Check sheet for the modelled part. Datum: model origin and axes. Units: mm. A direction names the side the tool comes from. Give positions to 0.01 mm unless a question says otherwise; leave off trailing zeros. Order: outer loops, then holes, each group sorted by start corner. A loop starts at its lowest first (then second) coordinate and runs counter-clockwise, first axis right, second up.
Item 1: Sectioned sample at C-C on z = 3.25. Record the boundary of the cut face in (x, y).
Item 2: Access from +Z, -Z, +X, -X, +Y, -Y to the whole of each face (thin tool, end or side, straight path). Record for faces 1 (the cylindrical face through (-1.952, 2.465, -1.864)), 2 (the flat face through (0, 6.35, 1)), 3 (the flat face through (1, 2.5, 2)).
Item 3: Sectioned sample at B-B on z = -1.43. Record the boundary of the cut face in (x, y), and give its area (3 significant figures).
Item 4: Material ranges on line 1 along X through (y, z) = (0.75, 0.75); line 2 along X through (y, z) = (2, -1.5); line 3 along X through (y, z) = (5.7, -1.43), recorded low to high.
Item 5: Sectioned sample at D-D on y = 3. Record the boundary of the cut face in (x, z).
Item 6: Gauge pin test, flat ends, axial feed: P1, Ø1.5, axis at x = -0.5, z = -0.5, coming from the -Y side; P2, Ø2.5, axis at x = 0, z = -1.43, coming from the -Y side. Record the tip position at first contact, or that the pin passes through.
Item 7: Sectioned sample at A-A on x = 0. Record the boundary of the cut face in (y, z), and give its area (3 significant figures).
Item 8: Release check for a two-part mould opening along X. For faces 4 (the flat face through (1.77, 1, 2)), 5 (the flat face through (2.16, 3, 0)), 6 (the flat face through (0, 0, 2)) record: released by +X, released by -X, zero draft, split by the parting line, or undercut.
from build123d import *

# Parameters (mm, degrees)
SKETCH_1_W          = 4.32
SKETCH_1_H          = 7.3
SKETCH_1_R          = 2
SKETCH_1_R_2        = 1.5
EXTRUDE_2_DEPTH     = 6.35
SKETCH_1_4_R        = 2
SKETCH_1_4_R_2      = 1.5
CUT_EXTRUDE_1_DEPTH = 5
SKETCH_2_W          = 1
SKETCH_2_H          = 4.148817955
CUT_EXTRUDE_2_DEPTH = 2.5


with BuildPart() as part:
    # Sketch 1 → Extrude 2 (new body)
    # profile 1 of 2: a face of its own
    with BuildSketch(Plane(origin=(0, 0, 0), x_dir=(1, 0, 0), z_dir=(0, 1, 0))):
        Rectangle(SKETCH_1_W, SKETCH_1_H)
        with Locations((0, 1.43)):
            Circle(SKETCH_1_R, mode=Mode.SUBTRACT)
    # profile 2 of 2: a face of its own
    with BuildSketch(Plane(origin=(0, 0, 0), x_dir=(1, 0, 0), z_dir=(0, 1, 0))):
        with Locations((0, 1.43)):
            Circle(SKETCH_1_R)
        with Locations(Location((0, 1.43, 0), (0, 0, 270))):
            Circle(SKETCH_1_R_2, mode=Mode.SUBTRACT)
    extrude(amount=EXTRUDE_2_DEPTH)

    # Sketch 1_4 → Cut-Extrude 1 (cut)
    with BuildSketch(Plane(origin=(0, 0, 0), x_dir=(1, 0, 0), z_dir=(0, 1, 0))):
        with Locations(Location((0, 1.43, 0), (0, 0, 270))):
            Circle(SKETCH_1_4_R)
        with Locations(Location((0, 1.43, 0), (0, 0, 270))):
            Circle(SKETCH_1_4_R_2, mode=Mode.SUBTRACT)
    extrude(amount=CUT_EXTRUDE_1_DEPTH, mode=Mode.SUBTRACT)

    # Sketch 2 → Cut-Extrude 2 (cut)
    with BuildSketch(Plane.XZ):
        with Locations((-1.27, 1.575591023)):
            Rectangle(SKETCH_2_W, SKETCH_2_H)
        with Locations((1.27, 1.575591023)):
            Rectangle(SKETCH_2_W, SKETCH_2_H)
    extrude(amount=-CUT_EXTRUDE_2_DEPTH, mode=Mode.SUBTRACT)


solid = part.part
Report:
1. outline: (-2.16, 0) - (-1.77, 0) - (-1.77, 2.5) - (-0.77, 2.5) - (-0.77, 0) - (0.77, 0) - (0.77, 2.5) - (1.77, 2.5) - (1.77, 0) - (2.16, 0) - (2.16, 6.35) - (-2.16, 6.35) - close
2. face 1: -Y
2. face 2: +Z, -Z, +X, -X, +Y
2. face 3: +Z, -Y
3. outline: (-2.16, 0) - (-2, 0) - (-2, 5) - (-1.5, 5) - (-1.5, 6.35) - (-2.16, 6.35) - close; (1.5, 5) - (2, 5) - (2, 0) - (2.16, 0) - (2.16, 6.35) - (1.5, 6.35) - close
3. area: 3.38 mm2
4. line 1: x = -2.16 to -1.77, -0.77 to 0.77, 1.77 to 2.16
4. line 2: x = -2.16 to -2, 2 to 2.16
4. line 3: x = -2.16 to -1.5, 1.5 to 2.16
5. outline: (-2.16, -3.65) - (2.16, -3.65) - (2.16, 3.65) - (-2.16, 3.65) - close; hole circle Ø4 at (0, -1.43)
6. P1: stops at y = 5
6. P2: passes through
7. outline: (0, -3.65) - (6.35, -3.65) - (6.35, -2.93) - (5, -2.93) - (5, -3.43) - (0, -3.43) - close; (0, 0.57) - (5, 0.57) - (5, 0.07) - (6.35, 0.07) - (6.35, 3.65) - (0, 3.65) - close
7. area: 22.3 mm2
8. face 4: undercut
8. face 5: released by +X
8. face 6: zero draft
